```python
from build123d import *
from build123d.topology import SkipClean

# Parameters (mm, degrees)
ESBO_O1_R                 = 1.65
RESSALTO_EXTRUS_O1_DEPTH  = 3
RESSALTO_EXTRUS_O2_START  = 15
ESBO_O2_R                 = 1.65
RESSALTO_EXTRUS_O2_DEPTH  = 15
CORTE_EXTRUS_O1_DEPTH     = 15
RESSALTO_EXTRUS_O3_DEPTH  = 2
ESBO_O6_W                 = 23.468316857
ESBO_O6_H                 = 21.298976644
CORTE_EXTRUS_O2_DEPTH     = 21
ESBO_O7_W                 = 18
ESBO_O7_H                 = 18
RESSALTO_EXTRUS_O4_DEPTH  = 2
CORTE_EXTRUS_O3_DEPTH     = 5
ESBO_O9_W                 = 18
ESBO_O9_H                 = 2
CORTE_EXTRUS_O4_DEPTH     = 8
ESBO_O10_W                = 18
ESBO_O10_H                = 12.25
RESSALTO_EXTRUS_O5_DEPTH  = 2
RESSALTO_EXTRUS_O6_DEPTH  = 5.85
ESBO_O12_W                = 2
ESBO_O12_H                = 2.6
RESSALTO_EXTRUS_O7_DEPTH  = 9.75
ESBO_O13_W                = 18
ESBO_O13_H                = 7.85
RESSALTO_EXTRUS_O8_DEPTH  = 1.5
ESBO_O14_W                = 18
ESBO_O14_H                = 1.5
RESSALTO_EXTRUS_O9_DEPTH  = 5.15
ESBO_O15_R                = 3.125
CORTE_EXTRUS_O5_DEPTH     = 5.15
ESBO_O16_W                = 2
ESBO_O16_H                = 2.625
RESSALTO_EXTRUS_O10_DEPTH = 5
ESBO_O18_W                = 2
ESBO_O18_H                = 2.6
RESSALTO_EXTRUS_O11_DEPTH = 5
ESBO_O19_W                = 18
ESBO_O19_H                = 2
RESSALTO_EXTRUS_O12_DEPTH = 5
ESBO_O20_W                = 18
ESBO_O20_H                = 1.5
RESSALTO_EXTRUS_O13_DEPTH = 5
ESBO_O21_W                = 18
ESBO_O21_H                = 7
RESSALTO_EXTRUS_O14_DEPTH = 3
ESBO_O22_W                = 18
ESBO_O22_H                = 2.75
RESSALTO_EXTRUS_O15_DEPTH = 9
ESBO_O23_W                = 18
ESBO_O23_H                = 3.006158343
RESSALTO_EXTRUS_O16_DEPTH = 6
ESBO_O24_W                = 27.560641217
ESBO_O24_H                = 36.557163592
CORTE_EXTRUS_O6_DEPTH     = 26
ESBO_O25_W                = 18
ESBO_O25_H                = 1.5
RESSALTO_EXTRUS_O17_DEPTH = 2
ESBO_O26_R                = 1.65
CORTE_EXTRUS_O7_DEPTH     = 10
FILETE1_R                 = 6
ESBO_O27_W                = 18
ESBO_O27_H                = 12.993841657
CORTE_EXTRUS_O8_DEPTH     = 1
ESBO_O28_W                = 18
ESBO_O28_H                = 9
RESSALTO_EXTRUS_O18_DEPTH = 1
ESBO_O29_W                = 2
ESBO_O29_H                = 2.6
CORTE_EXTRUS_O9_DEPTH     = 3


with BuildPart() as part:
    # Esboço1 → Ressalto-extrusão1 (new body)
    # profile 1 of 3: a face of its own
    with BuildSketch(Plane.XY):
        Polygon((-7, 15.25), (-9, 15.25), (-9, 13.25), (-9, 5), (-6.541451884, 0), (-2.020725942, -6), (2.020725942, -6), (6.541451884, 0), (9, 5), (9, 15.25), (7, 15.25), align=None)
        Polygon((2.020725942, -3.5), (4.041451884, 0), (2.020725942, 3.5), (-2.020725942, 3.5), (-4.041451884, 0), (-2.020725942, -3.5), align=None, mode=Mode.SUBTRACT)
        Polygon((-7, 13.25), (-7, 5), (0, 5), (7, 5), (7, 13.25), align=None, mode=Mode.SUBTRACT)
    # profile 2 of 3: a face of its own
    with BuildSketch(Plane.XY):
        Polygon((7, 13.25), (-7, 13.25), (-7, 5), (0, 5), (7, 5), align=None)
    # profile 3 of 3: a face of its own
    with BuildSketch(Plane.XY):
        Polygon((-2.020725942, -3.5), (2.020725942, -3.5), (4.041451884, 0), (2.020725942, 3.5), (-2.020725942, 3.5), (-4.041451884, 0), align=None)
        Circle(ESBO_O1_R, mode=Mode.SUBTRACT)
    extrude(amount=RESSALTO_EXTRUS_O1_DEPTH)

    # Esboço2 → Ressalto-extrusão2 (add)
    # profile 1 of 2: a face of its own
    with SkipClean():  # the faces are left unmerged after this step: merging them gives an invalid solid
        with BuildSketch(Plane(origin=(0, 0, 0), x_dir=(-1, 0, 0), z_dir=(0, 0, -1)).offset(RESSALTO_EXTRUS_O2_START)):
            Polygon((9, 5), (9, 15.25), (-9, 15.25), (-9, 5), (-6.541451884, 0), (-2.020725942, -6), (2.020725942, -6), (6.541451884, 0), align=None)
            Polygon((7, 5), (7, 13.25), (-7, 13.25), (-7, 5), (0, 5), align=None, mode=Mode.SUBTRACT)
            Polygon((-4.041451884, 0), (-2.020725942, -3.5), (2.020725942, -3.5), (4.041451884, 0), (2.020725942, 3.5), (-2.020725942, 3.5), align=None, mode=Mode.SUBTRACT)
        # profile 2 of 2: a face of its own
        with BuildSketch(Plane(origin=(0, 0, 0), x_dir=(-1, 0, 0), z_dir=(0, 0, -1)).offset(RESSALTO_EXTRUS_O2_START)):
            Polygon((-2.020725942, 3.5), (-4.041451884, 0), (-2.020725942, -3.5), (2.020725942, -3.5), (4.041451884, 0), (2.020725942, 3.5), align=None)
            Circle(ESBO_O2_R, mode=Mode.SUBTRACT)
        extrude(amount=-RESSALTO_EXTRUS_O2_DEPTH)

    # Esboço3 → Corte-extrusão1 (cut)
    with SkipClean():  # the faces are left unmerged after this step: merging them gives an invalid solid
        with BuildSketch(Plane(origin=(0, 0, -15), x_dir=(-1, 0, 0), z_dir=(0, 0, -1))):
            Polygon((-9, 10.625), (-9, 9.125), (-9, 7.625), (-7, 7.625), (-7, 10.625), align=None)
            Polygon((9, 7.625), (9, 9.125), (9, 10.625), (7, 10.625), (7, 7.625), align=None)
        extrude(amount=-CORTE_EXTRUS_O1_DEPTH, mode=Mode.SUBTRACT)

    # Esboço5 → Ressalto-extrusão3 (add)
    with SkipClean():  # the faces are left unmerged after this step: merging them gives an invalid solid
        with BuildSketch(Plane(origin=(0, 0, 0), x_dir=(-1, 0, 0), z_dir=(0, 0, -1))):
            Polygon((-1.583333333, 13.25), (-2.333333333, 13.25), (-3.083333333, 13.25), (-3.083333333, 5), (-1.583333333, 5), align=None)
        extrude(amount=RESSALTO_EXTRUS_O3_DEPTH)

    # Esboço6 → Corte-extrusão2 (cut)
    with BuildSketch(Plane(origin=(0, -16, 0), x_dir=(-1, 0, 0), z_dir=(0, -1, 0))):
        with Locations((-0.042259875, 5.70418088)):
            Rectangle(ESBO_O6_W, ESBO_O6_H)
    extrude(amount=-CORTE_EXTRUS_O2_DEPTH, mode=Mode.SUBTRACT)

    # Esboço7 → Ressalto-extrusão4 (add)
    with BuildSketch(Plane.XZ.offset(-5)):
        with Locations((0, -6)):
            Rectangle(ESBO_O7_W, ESBO_O7_H)
    extrude(amount=RESSALTO_EXTRUS_O4_DEPTH)

    # Esboço8 → Corte-extrusão3 (cut)
    with BuildSketch(Plane(origin=(0, 0, -15), x_dir=(-1, 0, 0), z_dir=(0, 0, -1))):
        Polygon((7, 7.625), (7, 5), (-7, 5), (-7, 7.625), (-9, 7.625), (-9, 3), (9, 3), (9, 7.625), align=None)
        Polygon((7, 10.625), (9, 10.625), (9, 15.25), (-9, 15.25), (-9, 10.625), (-7, 10.625), (-7, 13.25), (7, 13.25), align=None)
    extrude(amount=-CORTE_EXTRUS_O3_DEPTH, mode=Mode.SUBTRACT)

    # Esboço9 → Corte-extrusão4 (cut)
    with BuildSketch(Plane(origin=(0, 0, -10), x_dir=(-1, 0, 0), z_dir=(0, 0, -1))):
        with Locations((0, 14.25)):
            Rectangle(ESBO_O9_W, ESBO_O9_H)
    extrude(amount=-CORTE_EXTRUS_O4_DEPTH, mode=Mode.SUBTRACT)

    # Esboço24 → Corte-extrusão6 (cut)
    with BuildSketch(Plane.XY.offset(13)):
        with Locations((-1.631661855, 4.199263035)):
            Rectangle(ESBO_O24_W, ESBO_O24_H)
    extrude(amount=-CORTE_EXTRUS_O6_DEPTH, mode=Mode.SUBTRACT)


with BuildPart() as body_2:
    # Esboço10 → Ressalto-extrusão5 (new body)
    with BuildSketch(Plane(origin=(0, 0, -40), x_dir=(-1, 0, 0), z_dir=(0, 0, -1))):
        with Locations((0, 9.125)):
            Rectangle(ESBO_O10_W, ESBO_O10_H)
    extrude(amount=RESSALTO_EXTRUS_O5_DEPTH)

    # Esboço11 → Ressalto-extrusão6 (add)
    with BuildSketch(Plane.XY.offset(-40)):
        Polygon((9, 15.25), (-9, 15.25), (-9, 13.25), (-7, 13.25), (1.583333333, 13.25), (3.083333333, 13.25), (7, 13.25), (9, 13.25), align=None)
    extrude(amount=RESSALTO_EXTRUS_O6_DEPTH)

    # Esboço12 → Ressalto-extrusão7 (add)
    with BuildSketch(Plane.XY.offset(-40)):
        with Locations((8, 9.125)):
            Rectangle(ESBO_O12_W, ESBO_O12_H)
        with Locations((-8, 9.125)):
            Rectangle(ESBO_O12_W, ESBO_O12_H)
    extrude(amount=RESSALTO_EXTRUS_O7_DEPTH)

    # Esboço13 → Ressalto-extrusão8 (add)
    with BuildSketch(Plane(origin=(0, 15.25, 0), x_dir=(1, 0, 0), z_dir=(0, 1, 0))):
        with Locations((0, 38.075)):
            Rectangle(ESBO_O13_W, ESBO_O13_H)
    extrude(amount=RESSALTO_EXTRUS_O8_DEPTH)

    # Esboço14 → Ressalto-extrusão9 (add)
    with BuildSketch(Plane.XY.offset(-34.15)):
        with Locations((0, 16)):
            Rectangle(ESBO_O14_W, ESBO_O14_H)
    extrude(amount=RESSALTO_EXTRUS_O9_DEPTH)

    # Esboço15 → Corte-extrusão5 (cut)
    with BuildSketch(Plane(origin=(0, 0, -42), x_dir=(-1, 0, 0), z_dir=(0, 0, -1))):
        with Locations((0, 9.875)):
            Circle(ESBO_O15_R)
    extrude(amount=-CORTE_EXTRUS_O5_DEPTH, mode=Mode.SUBTRACT)

    # Esboço16 → Ressalto-extrusão10 (add)
    with BuildSketch(Plane.XY.offset(-40)):
        Polygon((-7, 7.625), (-9, 7.625), (-9, 3), (9, 3), (9, 7.625), (7, 7.625), (7, 5), (-7, 5), align=None)
        with Locations((-8, 11.9375)):
            Rectangle(ESBO_O16_W, ESBO_O16_H)
        with Locations((8, 11.9375)):
            Rectangle(ESBO_O16_W, ESBO_O16_H)
    extrude(amount=RESSALTO_EXTRUS_O10_DEPTH)

    # Esboço18 → Ressalto-extrusão11 (add)
    with BuildSketch(Plane.XY.offset(-30.25)):
        with Locations((-8, 9.125)):
            Rectangle(ESBO_O18_W, ESBO_O18_H)
        with Locations((8, 9.125)):
            Rectangle(ESBO_O18_W, ESBO_O18_H)
    extrude(amount=RESSALTO_EXTRUS_O11_DEPTH)

    # Esboço19 → Ressalto-extrusão12 (add)
    with BuildSketch(Plane.XY.offset(-34.15)):
        with Locations((0, 14.25)):
            Rectangle(ESBO_O19_W, ESBO_O19_H)
    extrude(amount=RESSALTO_EXTRUS_O12_DEPTH)

    # Esboço20 → Ressalto-extrusão13 (add)
    with BuildSketch(Plane.XY.offset(-29)):
        with Locations((0, 16)):
            Rectangle(ESBO_O20_W, ESBO_O20_H)
    extrude(amount=RESSALTO_EXTRUS_O13_DEPTH)

    # Esboço21 → Ressalto-extrusão14 (add)
    with BuildSketch(Plane.XZ.offset(-3)):
        with Locations((0, -38.5)):
            Rectangle(ESBO_O21_W, ESBO_O21_H)
    extrude(amount=RESSALTO_EXTRUS_O14_DEPTH)

    # Esboço22 → Ressalto-extrusão15 (add)
    with BuildSketch(Plane.XY.offset(-35)):
        with Locations((0, 1.375)):
            Rectangle(ESBO_O22_W, ESBO_O22_H)
    extrude(amount=RESSALTO_EXTRUS_O15_DEPTH)

    # Esboço23 → Ressalto-extrusão16 (add)
    with BuildSketch(Plane.XZ):
        with Locations((0, -27.503079172)):
            Rectangle(ESBO_O23_W, ESBO_O23_H)
    extrude(amount=RESSALTO_EXTRUS_O16_DEPTH)

    # Esboço25 → Ressalto-extrusão17 (add)
    with BuildSketch(Plane.XY.offset(-24)):
        with Locations((0, 16)):
            Rectangle(ESBO_O25_W, ESBO_O25_H)
    extrude(amount=RESSALTO_EXTRUS_O17_DEPTH)

    # Esboço26 → Corte-extrusão7 (cut)
    with BuildSketch(Plane(origin=(0, 0, -29.006158343), x_dir=(-1, 0, 0), z_dir=(0, 0, -1))):
        with Locations((0, -3)):
            Circle(ESBO_O26_R)
    extrude(amount=-CORTE_EXTRUS_O7_DEPTH, mode=Mode.SUBTRACT)

    # Filete1
    filete1_edges = [body_2.edges().sort_by_distance(p)[0] for p in [
        (-9, -6, -27.503079172),
        (9, -6, -27.503079172),
    ]]
    fillet(filete1_edges, radius=FILETE1_R)

    # Esboço27 → Corte-extrusão8 (cut)
    with BuildSketch(Plane.XZ):
        with Locations((0, -35.503079172)):
            Rectangle(ESBO_O27_W, ESBO_O27_H)
    extrude(amount=-CORTE_EXTRUS_O8_DEPTH, mode=Mode.SUBTRACT)

    # Esboço28 → Ressalto-extrusão18 (add)
    with BuildSketch(Plane(origin=(0, 2.75, 0), x_dir=(1, 0, 0), z_dir=(0, 1, 0))):
        with Locations((0, 30.5)):
            Rectangle(ESBO_O28_W, ESBO_O28_H)
    extrude(amount=RESSALTO_EXTRUS_O18_DEPTH)

    # Esboço29 → Corte-extrusão9 (cut)
    with BuildSketch(Plane.XY.offset(-25.25)):
        with Locations((8, 9.125)):
            Rectangle(ESBO_O29_W, ESBO_O29_H)
        with Locations((-8, 9.125)):
            Rectangle(ESBO_O29_W, ESBO_O29_H)
    extrude(amount=-CORTE_EXTRUS_O9_DEPTH, mode=Mode.SUBTRACT)


solid = body_2.part
```
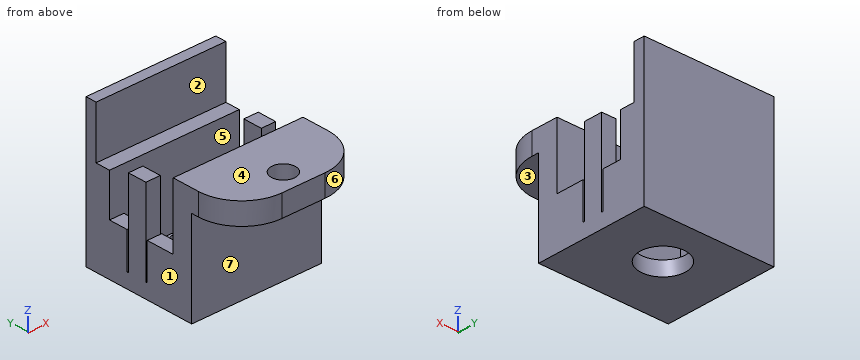
Work out the finished part from the listing and answer in its coordinate system (mm). Face numbers are marked on the shaded views. A direction names the side the tool comes from. Coordinates: 2 decimals unless noted, no trailing zeros. Loops run counter-clockwise (first coordinate to the right, second up) from the corner with the lowest first, then second, coordinate; pieces in that order, holes last. Notation, with made-up numbers: M 47,17 L 89,17 A12 ccw 89,35 Z; hole C -1,-17.5 d6. An arc over 180 degrees is marked long. Use CSV: the item, a comma, the result in double quotes. Start each with the question number.
(1) For the marked faces 1, 2, 3 and 4, determine the directions among +Z, -Z, +X, -X, +Y, -Y from which every point of the face is accessible in a straight line to the end or side of a thin tool.
(2) Find section B-B, the plane x = 0. Give the vertices of the cut face in (y, z), then the cut area to 3 significant figures.
(3) Consider line 1 (Y direction, x = 0, z = -40.65); line 2 (Y direction, x = 0, z = -28.1); line 3 (Y direction, x = -3.75, z = -39.5). Determine where each line is inside the solid, lowest interval first.
(4) For a pull along X with two mould halves and no side action, classify the marked faces 5, 6 and 7 as +X half, -X half, draft (parallel to the pull), parting line (faces both ways), or undercut.
(5) Find section A-A, the plane z = -31. Give the vertices of the cut face in (x, y) (3 decimals), then the cut area to 3 significant figures.
(6) Find section C-C, the plane y = -3. Give the vertices of the cut face in (x, z).
(7) Find section D-D, the plane z = -35.5. Give the vertices of the cut face in (x, y) (3 decimals), then the cut area to 3 significant figures.
(8) Given pin 1 Ø0.6 at (x, z) = (-7.5, -36.5) entering from -Y; pin 2 Ø10.5 at (x, y) = (-0.5, 0) entering from +Z; pin 3 Ø3 at (y, z) = (6, -26.5) entering from -X; pin 4 Ø1.6 at (x, y) = (-8, 12.5) entering from +Z, each flat-ended and moving along its own axis, determine where each tip first touches the part or whether it passes through.
Recorded:
1,face 1,"+Z, -Z, -X, +Y, -Y"
1,face 2,"+Z, +X, -X"
1,face 3,"-Z, +X, -X, -Y"
1,face 4,"+Z, +X, -X, -Y"
2,outline,"M -6,-29.01 L -4.65,-29.01 L -4.65,-26 L -6,-26 Z; M -1.35,-29.01 L 1,-29.01 L 1,-42 L 6.75,-42 L 6.75,-40 L 5,-40 L 5,-35 L 3.75,-35 L 3.75,-26 L -1.35,-26 Z; M 13,-42 L 16.75,-42 L 16.75,-22 L 15.25,-22 L 15.25,-29.15 L 13.25,-29.15 L 13.25,-40 L 13,-40 Z"
2,area,"124 mm^2"
3,line 1,"y = 1 to 6.75, 13 to 16.75"
3,line 2,"y = -6 to -4.65, -1.35 to 3.75, 15.25 to 16.75"
3,line 3,"y = 1 to 5, 13.25 to 16.75"
4,face 5,"undercut"
4,face 6,"+X half"
4,face 7,"draft"
5,outline,"M -9,1 L 9,1 L 9,3.75 L -9,3.75 Z; M -9,7.825 L -7,7.825 L -7,10.425 L -9,10.425 Z; M -9,13.25 L 9,13.25 L 9,16.75 L -9,16.75 Z; M 7,7.825 L 9,7.825 L 9,10.425 L 7,10.425 Z"
5,area,"123 mm^2"
6,outline,"M -8.2,-29.01 L -1.65,-29.01 L -1.65,-26 L -8.2,-26 Z; M 1.65,-29.01 L 8.2,-29.01 L 8.2,-26 L 1.65,-26 Z"
7,outline,"M -9,1 L 9,1 L 9,7.625 L 7,7.625 L 7,5 L -7,5 L -7,7.625 L -9,7.625 Z; M -9,7.825 L -7,7.825 L -7,10.425 L -9,10.425 Z; M -9,10.625 L -7,10.625 L -7,13.25 L 7,13.25 L 7,10.625 L 9,10.625 L 9,16.75 L -9,16.75 Z; M 7,7.825 L 9,7.825 L 9,10.425 L 7,10.425 Z"
7,area,"166 mm^2"
8,pin 1,"stops at y = 1"
8,pin 2,"stops at z = -26"
8,pin 3,"passes through"
8,pin 4,"stops at z = -29.15"
